Solid Edge part; units mm, degrees
sketch "Sketch1" plane through (0, 0, 0) normal (0, -1, 0) x (1, 0, 0)
  line L0 (29.5, 30) -> (29.5, 15)
  line L1 (-29.5, 15) -> (29.5, 15)
  line L2 (-29.5, 29) -> (-29.5, 15)
  line L3 (-29.5, 29) -> (22.7, 29)
  line L4 (22.7, 55) -> (22.7, 29)
  line L5 (27.5, 55) -> (22.7, 55)
  line L6 (27.5, 30) -> (27.5, 55)
  line L7 (27.5, 30) -> (29.5, 30)
  dimension "D1" = 29.5
  dimension "D2" = 27.5
  dimension "D3" = 27.5
  dimension "D4" = 27.5
  dimension "D5" = 29.5
  dimension "D6" = 29.5
revolve "RevolvedProtrusion1" add sketch "Sketch1" angle 360 about axis through (-60, 0, 0) along (1, 0, 0)
sketch "Sketch2" plane through (-29.5, 0, 0) normal (-1, 0, 0) x (0, -1, 0)
  line L0 (-4, 14) -> (4, 14)
  line L1 (4, 14) -> (4, 17)
  line L2 (4, 17) -> (-4, 17)
  line L3 (-4, 17) -> (-4, 14)
  dimension "D1" = 4
  dimension "D2" = 4
extrude "Cutout1" cut sketch "Sketch2" against normal through all
hole "Hole1" at (22.7, 0, 45) direction (1, 0, 0) diameter 8.4 end up to next
hole "Hole_5" at (0, -20.5061, -20.5061) direction (0, 0.7071, 0.7071) diameter 4.134 end up to next thread major 5 thread length 2
pattern_circular "Pattern1" count 6 over 360 about axis through (22.7, 0, 0) along (1, 0, 0) of "Hole1"
fillet "Round_1" radius 7 1 edges at (22.7, 0, -29)
fillet "Round_2" radius 7 1 edges at (-29.5, 0, -29)
properties material "Stainless steel"
Build history of the part. All positions in model axes, mm. A direction names the side the tool comes from. Round coordinates to 2 decimals unless told otherwise and drop trailing zeros. Write each loop counter-clockwise with the first axis right and the second up, starting at its lowest first coordinate (ties: lowest second). Pieces come first, ordered by that corner, then holes. Notation, with made-up numbers: (10.25, -29.5) - (21.25, -29.5) arc R11 cw to (21.25, -24.5) - close; hole circle Ø10 at (-24.5, 34). An arc over 180 degrees is marked (long way). Use CSV: the item, a comma, the result in double quotes.
(1) Band-saw the part on B-B (z = 0). Write the cut outline in (x, y).
Response:
outline,"(-29.5, -22) arc R7 ccw to (-22.5, -29) - (15.7, -29) arc R7 cw to (22.7, -36) - (22.7, -55) - (27.5, -55) - (27.5, -30) - (29.5, -30) - (29.5, -15) - (-29.5, -15) - close; (-29.5, 15) - (29.5, 15) - (29.5, 30) - (27.5, 30) - (27.5, 55) - (22.7, 55) - (22.7, 36) arc R7 cw to (15.7, 29) - (-22.5, 29) arc R7 ccw to (-29.5, 22) - close"
(2) 3-axis set-ups, long thin cutter, end or side, ignore diameter. For faces 4 (the cylindrical face through (-3.13, 25.73, 13.38)), 5 (the flat face through (29.5, -14, 6)), 6 (the flat face through (0, 4, 16)), 7 (the flat face through (27.5, 24, 24)): which of +Z, -Z, +X, -X, +Y, -Y reach the whole face in a straight line?
Response:
face 4,"-X"
face 5,"+Z, -Z, +X, +Y, -Y"
face 6,"+X, -X"
face 7,"+X"
(3) Band-saw the part on D-D (z = -45). Write the cut outline in (x, y), plus the area to 3 significant figures.
Response:
outline,"(22.7, -31.62) - (27.5, -31.62) - (27.5, -4.2) - (22.7, -4.2) - close; (22.7, 4.2) - (27.5, 4.2) - (27.5, 31.62) - (22.7, 31.62) - close"
area,"263 mm²"
(4) Band-saw the part on A-A (y = 0). Write the cut outline in (x, z).
Response:
outline,"(-29.5, -22) arc R7 ccw to (-22.5, -29) - (15.7, -29) arc R7 cw to (22.7, -36) - (22.7, -40.8) - (27.5, -40.8) - (27.5, -30) - (29.5, -30) - (29.5, -15) - (-29.5, -15) - close; (-29.5, 17) - (29.5, 17) - (29.5, 30) - (27.5, 30) - (27.5, 40.8) - (22.7, 40.8) - (22.7, 36) arc R7 cw to (15.7, 29) - (-22.5, 29) arc R7 ccw to (-29.5, 22) - close; (22.7, -55) - (27.5, -55) - (27.5, -49.2) - (22.7, -49.2) - close; (22.7, 49.2) - (27.5, 49.2) - (27.5, 55) - (22.7, 55) - close"
(5) Band-saw the part on C-C (x = -13). Write the cut outline in (y, z).
Response:
outline,"circle Ø58 at (0, 0); hole (-4, 14.46) arc R15 ccw (long way) to (4, 14.46) - (4, 17) - (-4, 17) - close"
(6) Pin check, flat tips, straight feed: P1, Ø8, axis at y = 27, z = 21, coming from the -X side; P2, Ø8, axis at x = 22, y = -15.5, coming from the +Z side; P3, Ø2, axis at y = -1, z = -40, coming from the +X side. Stop position of each tip, or through.
Response:
P1,"x = 19.63"
P2,"z = 53.77"
P3,"x = 27.5"
(7) Wall check: line 1 (Y direction, x = 25.75, z = 22.5); line 2 (X direction, y = -48, z = 11); line 3 (Z direction, x = 9, y = 0). Give the ranges that are in metal, low to high.
Response:
line 1,"-50.19 to -43.17, -34.77 to 34.77, 43.17 to 50.19"
line 2,"22.7 to 27.5"
line 3,"-29 to -15, 17 to 29"
(8) Mould opens along Y. For faces 1 (the cylindrical face through (25.066, -53.692, -11.923)), 2 (the flat face through (22.7, 36, 11)), 3 (the cylindrical face through (25.066, -1.262, -49.006)) say: pulls with the +Y half, pulls with the -Y half, needs draft (parallel to the pull), parting line crosses it, or undercut.
Response:
face 1,"parting line crosses it"
face 2,"needs draft"
face 3,"undercut"
